Source: CAD feature listing. Evaluate the final solid. Frame: model axes, mm. Coordinates: 2 decimals unless noted, no trailing zeros. Loops run counter-clockwise (first coordinate to the right, second up) from the corner with the lowest first, then second, coordinate; pieces in that order, holes last.
from build123d import *

# Parameters (mm, degrees)
SKETCH1_R           = 51.3588
BOSS_EXTRUDE1_DEPTH = 203.2
DOME1_FACE_RADIUS   = 51.3588
DOME1_HEIGHT        = 50.8


# Read off the part's stored shape, not the designer's step: Shell1
with BuildPart() as part:
    # Sketch1 → Boss-Extrude1 (new body)
    with BuildSketch(Plane(origin=(0, 0, 0), x_dir=(1, 0, 0), z_dir=(0, 1, 0))):
        with Locations(Location((0, 0, 0), (0, 0, 270))):
            Circle(SKETCH1_R)
    extrude(amount=BOSS_EXTRUDE1_DEPTH)

    # Dome1: a dome of height H over a round flat face of radius A is a cap of a sphere of radius (A * A + H * H) / (2 * H)
    dome1_r = (DOME1_FACE_RADIUS * DOME1_FACE_RADIUS + DOME1_HEIGHT * DOME1_HEIGHT) / (2 * DOME1_HEIGHT)
    dome1_base = Plane((0, 203.2, 0), z_dir=(0, 1, 0))
    with Locations(dome1_base.offset(DOME1_HEIGHT - dome1_r)):
        dome1_ball = Sphere(dome1_r, mode=Mode.PRIVATE)
    add(split(dome1_ball, bisect_by=dome1_base, keep=Keep.TOP, mode=Mode.PRIVATE))

    # Shell1 outline → Shell1 (revolve, cut)
    with BuildSketch(Plane.XY):
        with BuildLine():
            Line((50.8, 0), (50.800000001, 203.196935001))
            ThreePointArc((50.800000001, 203.196935001), (35.725082804, 238.75835259), (0, 253.4412))
            Line((0, 253.4412), (0, 0))
            Line((0, 0), (50.8, 0))
        make_face()
    revolve(axis=Axis((0, 0, 0), (0, 1, 0)), mode=Mode.SUBTRACT)


solid = part.part
Q1. Section A-A, the plane y = 109. Return the cut outline in (x, z).
Q2. Draft query along Z for faces 1 (the cylindrical face through (-45.564, 100.178, 23.699)), 2 (the flat face through (49.7, 0, -11.7)), 3 (the cylindrical face through (-11.012, 103.021, 49.592)). Return one class per face: +Z half, -Z half, draft (parallel to the pull), parting line (faces both ways), or undercut.
Q3. Contact query for flat-ended pins moving along their axis: pin 1 Ø12 at (y, z) = (213, 28.5) entering from -X; pin 2 Ø3 at (x, y) = (25, 177.5) entering from +Z; pin 3 Ø2 at (y, z) = (179, -39.5) entering from -X. Output: stop coordinate, or through.
Q4. Section D-D, the plane y = 235.5. Return the cut outline in (x, z).
Q5. Line query: line 1 along X through (y, z) = (176, 0); line 2 along Z through (x, y) = (-37, 97.5); line 3 along Z through (x, y) = (-33, 136). Output: solid intervals per line, ascending.
Derived:
1. outline: circle Ø102.72 at (0, 0); hole circle Ø101.6 at (0, 0)
2. face 1: parting line
2. face 2: draft
2. face 3: undercut
3. pin 1: stops at x = -45.24
3. pin 2: stops at z = 45.67
3. pin 3: stops at x = -33.99
4. outline: circle Ø78.95 at (0, 0); hole circle Ø77.49 at (0, 0)
5. line 1: x = -51.36 to -50.8, 50.8 to 51.36
5. line 2: z = -35.62 to -34.81, 34.81 to 35.62
5. line 3: z = -39.35 to -38.62, 38.62 to 39.35
